Can you work these out from the drawing? Everything is in mm from the part's minimum corner. Coordinates: 2 decimals unless noted, no trailing zeros. Order: outer loops, then holes, each group sorted by start corner. A loop starts at its lowest first (then second) coordinate and runs counter-clockwise, first axis right, second up. Notation, with made-up numbers: (87, 20) -> (136, 20) arc R12 cw to (136, 42) -> close; hole circle Ø9 at (-23, 76). An arc over 180 degrees is marked (long way). Answer in a Markdown table with one row per item.
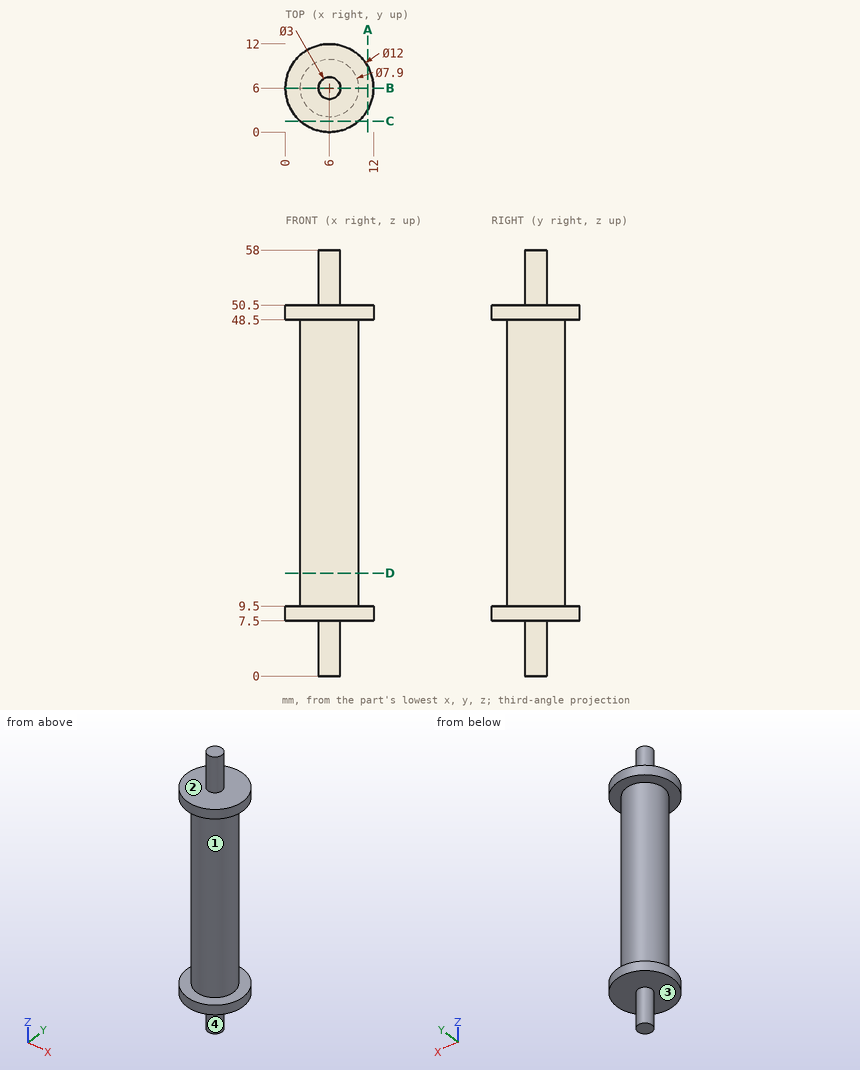
(1) I need wall thicknesses on line 1 (Z direction, x = 6.75, y = 11); line 2 (Z direction, x = 7, y = 8.75); line 3 (X direction, y = 9.25, z = 18) (3 decimals). Which ranges of each line are inside material? Lowest first, please. Write a range as [from, to].
Response values:
| item | result |
|---|---|
| line 1 | [7.5, 9.5], [48.5, 50.5] |
| line 2 | [7.5, 50.5] |
| line 3 | [3.755, 8.245] |
(2) Suppose I cut it at B-B (y = 6). Please give me the cut outline in (x, z), and give its area (3 significant figures).
Response values:
| item | result |
|---|---|
| outline | (0, 7.5) -> (4.5, 7.5) -> (4.5, 0) -> (7.5, 0) -> (7.5, 7.5) -> (12, 7.5) -> (12, 9.5) -> (9.95, 9.5) -> (9.95, 48.5) -> (12, 48.5) -> (12, 50.5) -> (7.5, 50.5) -> (7.5, 58) -> (4.5, 58) -> (4.5, 50.5) -> (0, 50.5) -> (0, 48.5) -> (2.05, 48.5) -> (2.05, 9.5) -> (0, 9.5) -> close |
| area | 401 mm2 |
(3) We'd pull the mould along Z, two halves only. Please class the marked faces 1, 2, 3 and 4: +Z half, -Z half, draft (parallel to the pull), parting line (faces both ways), or undercut.
Response values:
| item | result |
|---|---|
| face 1 | undercut |
| face 2 | +Z half |
| face 3 | -Z half |
| face 4 | draft |
(4) Suppose I cut it at A-A (x = 11.25). Please give me the cut outline in (y, z).
Response values:
| item | result |
|---|---|
| outline | (3.1, 7.5) -> (8.9, 7.5) -> (8.9, 9.5) -> (3.1, 9.5) -> close; (3.1, 48.5) -> (8.9, 48.5) -> (8.9, 50.5) -> (3.1, 50.5) -> close |
(5) Suppose I cut it at D-D (z = 14). Please give me the cut outline in (x, y).
Response values:
| item | result |
|---|---|
| outline | circle Ø7.9 at (6, 6) |
(6) Will these pins go through, and if not, where does the flat tip stop? pin 1 Ø4 at (x, y) = (1.5, 8) entering from +Z; pin 2 Ø6 at (x, y) = (4.5, 10.5) entering from -Z; pin 3 Ø1 at (y, z) = (4.5, 34) entering from -X.
Response values:
| item | result |
|---|---|
| pin 1 | z = 50.5 |
| pin 2 | z = 7.5 |
| pin 3 | x = 2.18 |
(7) Suppose I cut it at C-C (y = 1.5). Please give me the cut outline in (x, z), and give its area (3 significant figures).
Response values:
| item | result |
|---|---|
| outline | (2.03, 7.5) -> (9.97, 7.5) -> (9.97, 9.5) -> (2.03, 9.5) -> close; (2.03, 48.5) -> (9.97, 48.5) -> (9.97, 50.5) -> (2.03, 50.5) -> close |
| area | 31.7 mm2 |
